Drawing for the job (mm, zero at the part's lowest x, y, z). A direction names the side the tool comes from. Give positions to 0.01 mm unless a question says otherwise; leave off trailing zeros. Order: outer loops, then holes, each group sorted by start corner. A loop starts at its lowest first (then second) coordinate and runs counter-clockwise, first axis right, second up. Notation, with made-up numbers: (-10.75, -7.75) - (12.25, -7.75) arc R21 ccw to (12.25, 16.25) - close; hole circle Ø1 at (-39.75, 33.5). An arc over 180 degrees is marked (long way). Use a Markdown table: item, result.
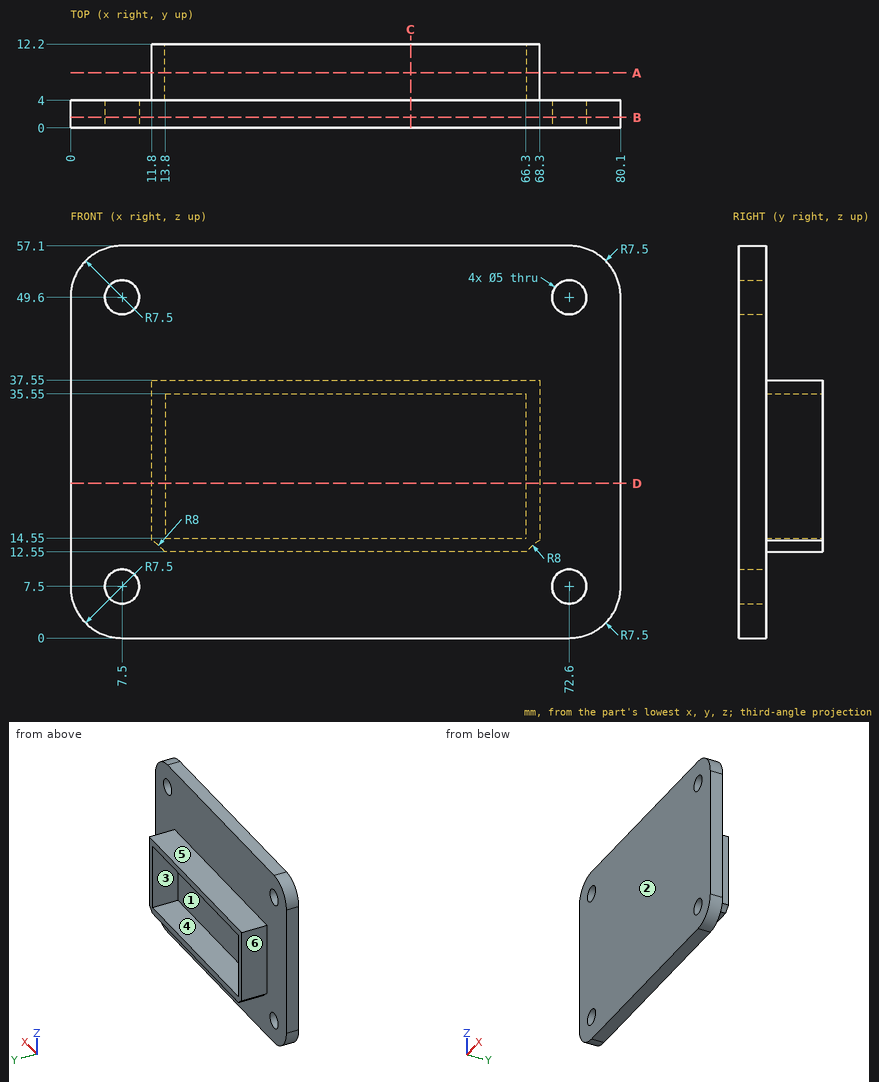
1) Slice it at D-D (z = 22.5). Write the cut outline in (x, y).
Computed:
| item | result |
|---|---|
| outline | (0, 0) - (80.1, 0) - (80.1, 4) - (68.3, 4) - (68.3, 12.2) - (66.3, 12.2) - (66.3, 4) - (13.8, 4) - (13.8, 12.2) - (11.8, 12.2) - (11.8, 4) - (0, 4) - close |
2) Slice it at B-B (y = 1.5). Write the cut outline in (x, z).
Computed:
| item | result |
|---|---|
| outline | (0, 7.5) arc R7.5 ccw to (7.5, 0) - (72.6, 0) arc R7.5 ccw to (80.1, 7.5) - (80.1, 49.6) arc R7.5 ccw to (72.6, 57.1) - (7.5, 57.1) arc R7.5 ccw to (0, 49.6) - close; hole circle Ø5 at (7.5, 7.5); hole circle Ø5 at (7.5, 49.6); hole circle Ø5 at (72.6, 7.5); hole circle Ø5 at (72.6, 49.6) |
3) Two-plate mould, pull along Z, no slides. Class the marked faces 3, 4, 5 and 6: +Z half, -Z half, draft (parallel to the pull), parting line (faces both ways), or undercut.
Computed:
| item | result |
|---|---|
| face 3 | undercut |
| face 4 | undercut |
| face 5 | +Z half |
| face 6 | draft |
4) Slice it at A-A (y = 8). Write the cut outline in (x, z).
Computed:
| item | result |
|---|---|
| outline | (11.8, 14.25) arc R8 cw to (13.7, 12.55) - (66.4, 12.55) arc R8 cw to (68.3, 14.25) - (68.3, 37.55) - (11.8, 37.55) - close; hole (13.8, 14.55) - (66.3, 14.55) - (66.3, 35.55) - (13.8, 35.55) - close |
5) Pin check, flat tips, straight feed: P1, Ø6.5, axis at y = 7, z = 26, coming from the -X side; P2, Ø3, axis at y = 7, z = 50, coming from the -X side; P3, Ø6.5, axis at x = 7.5, z = 7.5, coming from the +Y side; P4, Ø4, axis at y = 9, z = 22.5, coming from the +X side. Stop position of each tip, or through.
Computed:
| item | result |
|---|---|
| P1 | stops at x = 0 |
| P2 | passes through |
| P3 | stops at y = 4 |
| P4 | stops at x = 68.3 |
6) Tool access for the marked faces 1 and 2: list every direction of +Z, -Z, +X, -X, +Y, -Y with a clear straight run to the whole face (end or side of a thin tool).
Computed:
| item | result |
|---|---|
| face 1 | +Y |
| face 2 | +Z, -Z, +X, -X, -Y |
7) Slice it at C-C (x = 49.5). Write the cut outline in (y, z).
Computed:
| item | result |
|---|---|
| outline | (0, 0) - (4, 0) - (4, 12.55) - (12.2, 12.55) - (12.2, 14.55) - (4, 14.55) - (4, 35.55) - (12.2, 35.55) - (12.2, 37.55) - (4, 37.55) - (4, 57.1) - (0, 57.1) - close |
8) Wall check: line 1 (Z direction, x = 72.6, y = 1); line 2 (Z direction, x = 24, y = 5.75); line 3 (Y direction, x = 24, z = 23). Give the ranges that are in metal, low to high. Write a range as from..to.
Computed:
| item | result |
|---|---|
| line 1 | z = 0..5, 10..47.1, 52.1..57.1 |
| line 2 | z = 12.55..14.55, 35.55..37.55 |
| line 3 | y = 0..4 |
